Check sheet for the modelled part. Datum: model origin and axes. Units: mm. A direction names the side the tool comes from. Round coordinates to 2 decimals unless told otherwise and drop trailing zeros. Write each loop counter-clockwise with the first axis right and the second up, starting at its lowest first coordinate (ties: lowest second). Pieces come first, ordered by that corner, then holes. Notation, with made-up numbers: (23.5, -9) -> (47.5, -9) arc R27 ccw to (47.5, 25) -> close; hole circle Ø4 at (-16.5, 3). An arc over 180 degrees is marked (long way). One line per item, written item: value.
from build123d import *

# Parameters (mm, degrees)
SKETCH006_W  = 5.4
SKETCH006_H  = 5.4
PAD003_DEPTH = 3
SKETCH007_W  = 5.8
SKETCH007_H  = 5.8
PAD004_DEPTH = 1
SKETCH008_R  = 1.25
PAD005_DEPTH = 2


with BuildPart() as part:
    # Sketch006 → Pad003 (new body)
    with BuildSketch(Plane.XY):
        with Locations((15.2, 19)):
            Rectangle(SKETCH006_W, SKETCH006_H)
    extrude(amount=PAD003_DEPTH)

    # Sketch007 → Pad004 (join)
    with BuildSketch(Plane.XY):
        with Locations((15.2, 19)):
            Rectangle(SKETCH007_W, SKETCH007_H)
    extrude(amount=PAD004_DEPTH)

    # Sketch008 → Pad005 (join)
    with BuildSketch(Plane.XY):
        with Locations((15.2, 19)):
            Circle(SKETCH008_R)
    extrude(amount=-PAD005_DEPTH)


with BuildPart() as part_1:
    # Body003 placement: moved
    add(part.part.moved(Location((0, 0, 8.5))))


solid = part_1.part
Item 1: Sectioned sample at C-C on z = 6.9. Enter the section's corners in (x, y), and give its area (3 significant figures).
Answer:
outline: circle Ø2.5 at (15.2, 19)
area: 4.91 mm^2
Item 2: Sectioned sample at D-D on x = 15.2. Enter the section's corners in (y, z).
Answer:
outline: (16.1, 8.5) -> (17.75, 8.5) -> (17.75, 6.5) -> (20.25, 6.5) -> (20.25, 8.5) -> (21.9, 8.5) -> (21.9, 9.5) -> (21.7, 9.5) -> (21.7, 11.5) -> (16.3, 11.5) -> (16.3, 9.5) -> (16.1, 9.5) -> close
Item 3: Depth check by flat-ended pin: P1, Ø2, axis at x = 14, z = 11, coming from the -Y side; P2, Ø1.5, axis at y = 20, z = 7.5, coming from the +X side; P3, Ø0.6, axis at y = 18.5, z = 10.5, coming from the -X side. Enter the tip coordinate at first touch or a pass-through.
Answer:
P1: stops at y = 16.3
P2: stops at x = 16.42
P3: stops at x = 12.5
Item 4: Sectioned sample at A-A on x = 12.85. Enter the section's corners in (y, z).
Answer:
outline: (16.1, 8.5) -> (21.9, 8.5) -> (21.9, 9.5) -> (21.7, 9.5) -> (21.7, 11.5) -> (16.3, 11.5) -> (16.3, 9.5) -> (16.1, 9.5) -> close
Item 5: Tool access check on faces 1 (the flat face through (15, 21.7, 10)), 2 (the cylindrical face through (14.93, 17.78, 7.51)), 3 (the flat face through (17.9, 19, 10)), 4 (the flat face through (12.5, 19, 10)), 5 (the flat face through (15, 16.3, 10)). Record the directions out of +Z, -Z, +X, -X, +Y, -Y that give a thin tool (end or side, any length) a straight path to the whole face; none if there is none.
Answer:
face 1: +Z, +X, -X, +Y
face 2: -Z
face 3: +Z, +X, +Y, -Y
face 4: +Z, -X, +Y, -Y
face 5: +Z, +X, -X, -Y
Item 6: Sectioned sample at B-B on y = 19. Enter the section's corners in (x, z).
Answer:
outline: (12.3, 8.5) -> (13.95, 8.5) -> (13.95, 6.5) -> (16.45, 6.5) -> (16.45, 8.5) -> (18.1, 8.5) -> (18.1, 9.5) -> (17.9, 9.5) -> (17.9, 11.5) -> (12.5, 11.5) -> (12.5, 9.5) -> (12.3, 9.5) -> close
Item 7: Thickness scan on line 1 (Z direction, x = 17.75, y = 19.95); line 2 (X direction, y = 21.35, z = 10.6); line 3 (Y direction, x = 13.9, z = 10). Record the ranges inside material, lowest first.
Answer:
line 1: z = 8.5 to 11.5
line 2: x = 12.5 to 17.9
line 3: y = 16.3 to 21.7
